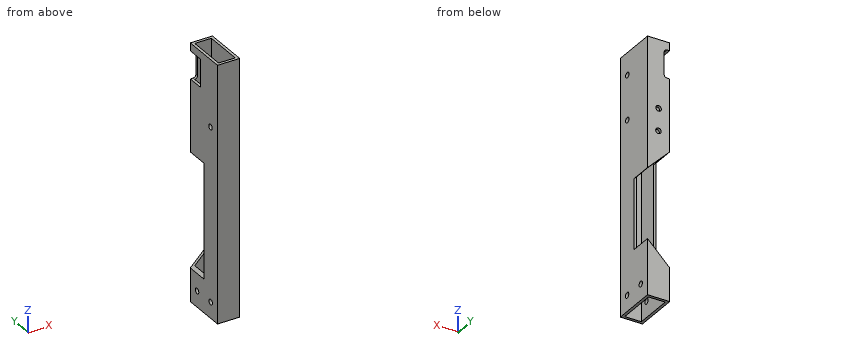
Autodesk Inventor part; units mm, degrees
ref_plane "YZ Plane" through (0, 0, 0) normal (1, 0, 0) x (0, 1, 0)
ref_plane "XZ Plane" through (0, 0, 0) normal (0, 1, 0) x (-1, 0, 0)
ref_plane "XY Plane" through (0, 0, 0) normal (0, 0, 1) x (1, 0, 0)
sketch "Sketch1" plane through (0, 0, 0) normal (0, 0, 1) x (1, 0, 0)
  line L0 (0, 0) -> (25.4, 0)
  line L1 (25.4, 0) -> (25.4, 50.8)
  line L2 (25.4, 50.8) -> (0, 50.8)
  line L3 (0, 50.8) -> (0, 0)
  line L4 (3.175, 47.625) -> (22.225, 47.625)
  line L5 (22.225, 47.625) -> (22.225, 3.175)
  line L6 (22.225, 3.175) -> (3.175, 3.175)
  line L7 (3.175, 3.175) -> (3.175, 47.625)
  dimension "d0" = 25.4
  dimension "d1" = 50.8
  dimension "d2" = 3.175
extrude "Extrusion1" add sketch "Sketch1" along normal blind 292.1
sketch "Sketch2" plane through (0, 50.8, 0) normal (0, 1, 0) x (1, 0, 0)
  line L0 (25.4, 0) -> (25.4, -292.1)
  line L1 (0, 0) -> (0, -292.1)
  line L2 (25.4, -63.4492) -> (0, -38.0492)
  line L3 (25.4, -143.5862) -> (0, -168.9862)
  line L4 (0, -168.9862) -> (0, -38.0492)
  line L5 (25.4, -143.5862) -> (25.4, -63.4492)
extrude "Extrusion2" cut sketch "Sketch2" against normal blind 25.4
sketch "Sketch3" plane through (25.4, 0, 0) normal (1, 0, 0) x (0, 0, -1)
  line L0 (-15.2442, 1673.225) -> (-15.2442, -149.225)
  line L1 (17.7758, 1673.225) -> (17.7758, -149.225)
  circle A0 centre (-215.7344, 12.9914) radius 3.175
  circle A1 centre (-14.559, 38.1) radius 3.175
  circle A2 centre (-14.559, 12.7) radius 3.175
  line L2 (-34.8742, 50.8) -> (-34.8742, 25.4)
  line L3 (-34.8742, 25.4) -> (-169.9072, 25.4)
  line L4 (-169.9072, 25.4) -> (-169.9072, 50.8)
  line L5 (-169.9072, 50.8) -> (-234.7144, 50.8)
  line L6 (-234.7144, 50.8) -> (-234.7144, 0)
  line L7 (0, 0) -> (-234.7144, 0)
  line L8 (0, 50.8) -> (0, 0)
  line L9 (0, 50.8) -> (-34.8742, 50.8)
  line L10 (0, 0) -> (-292.1, 0)
  line L11 (-34.8742, 50.8) -> (17.7758, 50.8)
  line L12 (17.7758, 50.8) -> (17.7758, 0)
  line L13 (17.7758, 0) -> (-34.8742, 0)
  line L14 (-34.8742, 0) -> (-34.8742, 50.8)
  circle A3 centre (-18.3666, 38.1) radius 3.175
  circle A4 centre (-18.3666, 12.7) radius 3.175
  dimension "d7" = 6.35
  dimension "d8" = 6.35
extrude "Extrusion3" cut sketch "Sketch3" against normal blind 25.4 contours A3 L0 | L0 A3 A1 | A1 A3 | A4 L0 | L0 A4 A2 | A2 A4 picked at (-16.0741, 38.1) picked at (-16.0741, 12.7)
sketch "Sketch4" plane through (0, 50.8, 292.1) normal (0, 1, 0) x (1, 0, 0)
  circle A0 centre (12.7528, 77.8097) radius 3.175
  circle A1 centre (-65.5643, -12.7) radius 3.175
  circle A2 centre (16.4357, -12.7) radius 3.175
  circle A3 centre (-65.5643, 77.8097) radius 3.175
  line L0 (-75.3643, -25.3975) -> (26.2357, -25.3975)
  line L1 (26.2357, 88.0643) -> (26.2357, -25.3975)
  line L2 (26.2357, 88.0643) -> (-75.3643, 88.0643)
  line L3 (-75.3643, 88.0643) -> (-75.3643, -25.3975)
  circle A4 centre (-24.5643, 24.5643) radius 41
  circle A5 centre (-24.6714, 70.0642) radius 2.55
  circle A6 centre (-70.0642, 24.4572) radius 2.55
  circle A7 centre (-24.4572, -20.9355) radius 2.55
  circle A8 centre (20.9355, 24.6714) radius 2.55
  circle A9 centre (7.5332, 56.8133) radius 2.55
  circle A10 centre (7.6847, -7.5332) radius 2.55
  circle A11 centre (-56.6619, -7.6847) radius 2.55
  circle A12 centre (-56.8133, 56.6619) radius 2.55
  circle A13 centre (-65.5643, 77.8097) radius 3.175
  circle A14 centre (-65.5643, -12.7) radius 3.175
  circle A15 centre (16.4357, -12.7) radius 3.175
  circle A16 centre (-24.5643, 24.5643) radius 9.525
  circle A17 centre (12.9268, 103.2097) radius 3.175
  circle A18 centre (-78.1301, -12.7) radius 3.175
  circle A19 centre (12.7528, 77.8097) radius 3.175
  line L4 (25.4, -25.4) -> (-88.9, -25.4)
  line L5 (25.4, 123.9554) -> (25.4, -25.4)
  line L6 (25.4, 123.9554) -> (-88.9, 92.2721)
  line L7 (-88.9, -25.4) -> (-88.9, 92.2721)
  point P0 (0, 292.1)
extrude "Extrusion4" cut sketch "Sketch4" against normal blind 25.4 contours A0 | A17
sketch "Sketch5" plane through (25.4, 0, 0) normal (1, 0, 0) x (0, 0, -1)
  line L0 (-292.1, 0) -> (-292.1, 50.8)
  line L1 (0, 0) -> (-292.1, 0)
  point P0 (-266.7, 13.081)
  point P1 (-215.9, 13.081)
  dimension "d13" = 25.4
  dimension "d14" = 50.8
  dimension "d15" = 13.081
  dimension "d16" = 13.081
hole "Hole1" at (25.4, 13.081, 266.7) at (25.4, 13.081, 215.9) direction (-1, 0, 0) diameter 6.35 end through all
sketch "Sketch6" plane through (0, 0, 0) normal (0, -1, 0) x (1, 0, 0)
  circle A0 centre (-24.5643, 267.5357) radius 28.3845
  point P0 (0, 0)
extrude "Extrusion5" cut sketch "Sketch6" against normal blind 50.8
sketch "Sketch7" plane through (0, 50.8, 292.1) normal (0, 1, 0) x (1, 0, 0)
  line L0 (0, 10.3421) -> (0, 0)
  line L1 (0, 8.9261) -> (6.3676, 8.9261)
  line L2 (6.3676, 8.9261) -> (6.3676, 40.6761)
  line L3 (6.3676, 40.6761) -> (0, 40.6761)
  line L4 (0, 40.6761) -> (0, 8.9261)
  point P0 (0, 292.1)
  dimension "d26" = 31.75
extrude "Extrusion6" cut sketch "Sketch7" against normal blind 19.05
fillet "Fillet1" radius 3.175 1 edges at (6.3676, 49.2125, 251.4239)
fillet "Fillet2" radius 3.175 1 edges at (6.3676, 49.2125, 283.1739)
sketch "Sketch8" plane through (0, 0, 0) normal (0, -1, 0) x (1, 0, 0)
  line L0 (0, 283.1739) -> (0, 292.1)
  line L1 (3.175, 165.8112) -> (3.175, 251.4239)
  line L2 (0, 284.5553) -> (3.175, 284.5553)
  line L3 (3.175, 284.5553) -> (3.175, 247.1802)
  line L4 (3.175, 247.1802) -> (0, 247.1802)
  line L5 (0, 247.1802) -> (0, 284.5553)
  point P0 (0, 0)
extrude "Extrusion7" add sketch "Sketch8" against normal blind 31.75
sketch "Sketch9" plane through (0, 0, 0) normal (0, -1, 0) x (1, 0, 0)
  line L0 (1.5802, 280.6086) -> (8.0596, 280.6086)
  line L1 (8.0596, 280.6086) -> (8.0596, 250.8034)
  line L2 (8.0596, 250.8034) -> (1.5802, 250.8034)
  line L3 (1.5802, 250.8034) -> (1.5802, 280.6086)
  point P0 (0, 0)
extrude "Extrusion8" add sketch "Sketch9" against normal blind 3.175
properties part number "Fender Side Right"
Verification items for the finished model (mm, model axes). Round coordinates to 2 decimals unless told otherwise and drop trailing zeros. Order: outer loops, then holes, each group sorted by start corner. A loop starts at its lowest first (then second) coordinate and runs counter-clockwise, first axis right, second up.
1) Cross-section at D-D, the plane z = 80.5. Record the cut outline in (x, y) (3 decimals), plus the area to 3 significant figures.
Geometry says:
outline: (0, 0) - (25.4, 0) - (25.4, 25.4) - (22.225, 25.4) - (22.225, 3.175) - (3.175, 3.175) - (3.175, 25.4) - (0, 25.4) - close
area: 222 mm2
2) Cross-section at A-A, the plane y = 23. Record the cut outline in (x, z) (3 decimals).
Geometry says:
outline: (0, 0) - (3.175, 0) - (3.175, 292.1) - (0, 292.1) - close; (22.225, 0) - (25.4, 0) - (25.4, 292.1) - (22.225, 292.1) - close
3) Cross-section at C-C, the plane x = 19.5. Record the cut outline in (y, z) (3 decimals).
Geometry says:
outline: (0, 0) - (3.175, 0) - (3.175, 292.1) - (0, 292.1) - close; (47.625, 0) - (50.8, 0) - (50.8, 57.549) - (47.625, 57.549) - close; (47.625, 149.486) - (50.8, 149.486) - (50.8, 292.1) - (47.625, 292.1) - close
4) Depth check by flat-ended pin: pin 1 (4 mm diameter, centred on x = 20, y = 41.5, fed in from -Z); pin 2 (2.5 mm diameter, centred on x = 24, z = 120.5, fed in from +Y); pin 3 (6 mm diameter, centred on x = 16.5, z = 77.5, fed in from +Y) (3 decimals). Enter the tip coordinate at first touch or a pass-through.
Geometry says:
pin 1: passes through
pin 2: stops at y = 25.4
pin 3: stops at y = 3.175
5) Cross-section at B-B, the plane z = 266.7. Record the cut outline in (x, y) (3 decimals).
Geometry says:
outline: (0, 0) - (25.4, 0) - (25.4, 9.906) - (22.225, 9.906) - (22.225, 3.175) - (3.175, 3.175) - (3.175, 31.75) - (0, 31.75) - close; (6.368, 47.625) - (22.225, 47.625) - (22.225, 16.256) - (25.4, 16.256) - (25.4, 50.8) - (6.368, 50.8) - close
6) Material ranges on line 1 (X direction, y = 3.5, z = 273.5) (3 decimals); line 2 (Y direction, x = 23.15, z = 215.9); line 3 (Z direction, x = 23.95, y = 12.7), recorded low to high.
Geometry says:
line 1: x = 0 to 3.175, 22.225 to 25.4
line 2: y = 0 to 9.91, 16.26 to 50.8
line 3: z = 0 to 15.19, 21.54 to 212.75, 219.05 to 263.55, 269.85 to 292.1
